from build123d import *

# Parameters (mm, degrees)
EXTRUDE_START       = 40
EXTRUDE_1_DEPTH     = 460
SKETCH_2_W          = 13.894074778
SKETCH_2_H          = 174.961932369
CUT_EXTRUDE_1_DEPTH = 501.611575003


with BuildPart() as part:
    # Эскиз1 → Вытянуть1 (new body)
    with BuildSketch(Plane(origin=(0, 0, 0), x_dir=(1, 0, 0), z_dir=(0, 1, 0)).offset(EXTRUDE_START)):
        with BuildLine():
            Line((-17.766709847, 14.4460477), (-16.308397656, 15.700046652))
            Line((-16.308397656, 15.700046652), (-4.722880617, 2.226908794))
            ThreePointArc((-4.722880617, 2.226908794), (-3.017444081, 0.942662024), (-0.931762463, 0.48688167))
            Line((-0.931762463, 0.48688167), (17.122829042, 0.48688167))
            Line((17.122829042, 0.48688167), (17.122829042, -1.51311833))
            Line((17.122829042, -1.51311833), (-4.043463493, -1.51311833))
            Line((-4.043463493, -1.51311833), (-17.766709847, 14.4460477))
        make_face()
    extrude(amount=EXTRUDE_1_DEPTH)

    # Эскиз2 → Вырез-Вытянуть1 (cut, through all)
    with BuildSketch(Plane.XY.offset(1.51311833)):
        with Locations((12.875765805, 223.422280108)):
            Rectangle(SKETCH_2_W, SKETCH_2_H)
    extrude(amount=-CUT_EXTRUDE_1_DEPTH, mode=Mode.SUBTRACT)


solid = part.part
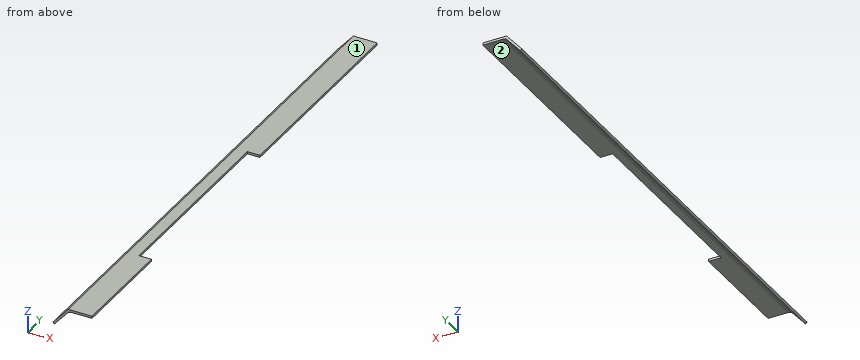
Check sheet for the modelled part. Datum: model origin and axes. Units: mm. Face numbers are marked on the shaded views. A direction names the side the tool comes from. Round coordinates to 2 decimals unless told otherwise and drop trailing zeros. Write each loop counter-clockwise with the first axis right and the second up, starting at its lowest first coordinate (ties: lowest second). Pieces come first, ordered by that corner, then holes. Notation, with made-up numbers: (-27, 5) - (5, 5) arc R10 cw to (5, 18) - close; hole circle Ø5 at (-37, 4.25). An arc over 180 degrees is marked (long way). Return JSON: item names as keys, results as strings.
Q1. Depth check by flat-ended pin: P1, Ø3, axis at y = 365, z = -12.5, coming from the -X side; P2, Ø14.5, axis at x = 8.5, y = 313.5, coming from the -Z side; P3, Ø3, axis at x = 8, y = 299.5, coming from the +Z side; P4, Ø0.6, axis at y = 194, z = 0.5, coming from the +X side. Enter the tip coordinate at first touch or a pass-through.
Returned:
{"P1": "stops at x = -17.38", "P2": "stops at z = -0.49", "P3": "passes through", "P4": "stops at x = 5.93"}
Q2. Scan lines: L1, parallel to Z at x = 8, y = 419; L2, parallel to Y at x = 13, z = -0.25; L3, parallel to X at y = 78, z = -10. Record each from-to range of solid material in increasing order. Write a range as from..to.
Returned:
{"L1": "z = -0.49..1.51", "L2": "y = 40..135.94, 310.9..500", "L3": "x = -13.94..-11.41"}
Q3. Cross-section at A-A (x = 10). Record the boundary of the cut face in (y, z), then the cut area to 3 significant figures.
Returned:
{"outline": "(40, -0.49) - (135.94, -0.49) - (135.94, 1.51) - (40, 1.51) - close; (310.9, -0.49) - (500, -0.49) - (500, 1.51) - (310.9, 1.51) - close", "area": "570 mm²"}
Q4. Cross-section at C-C (y = 321). Record the boundary of the cut face in (x, z), then the cut area to 3 significant figures.
Returned:
{"outline": "(-17.77, -14.45) - (-16.31, -15.7) - (-4.72, -2.23) arc R5 cw to (-0.93, -0.49) - (17.12, -0.49) - (17.12, 1.51) - (-4.04, 1.51) - close", "area": "81.8 mm²"}
Q5. Cross-section at B-B (y = 275). Record the boundary of the cut face in (x, z), then the cut area to 3 significant figures.
Returned:
{"outline": "(-17.77, -14.45) - (-16.31, -15.7) - (-4.72, -2.23) arc R5 cw to (-0.93, -0.49) - (5.93, -0.49) - (5.93, 1.51) - (-4.04, 1.51) - close", "area": "59.4 mm²"}
Q6. Access from +Z, -Z, +X, -X, +Y, -Y to the whole of each face (thin tool, end or side, straight path). Record for the marked faces 1 and 2.
Returned:
{"face 1": "+Z, +X, -X, +Y, -Y", "face 2": "-Z, +X, +Y, -Y"}
Q7. Cross-section at D-D (z = -9.5). Record the boundary of the cut face in (x, y).
Returned:
{"outline": "(-13.51, 40) - (-10.98, 40) - (-10.98, 500) - (-13.51, 500) - close"}
